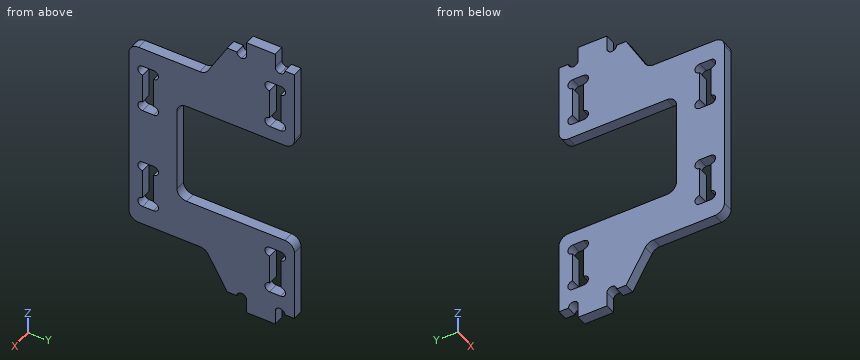
from build123d import *

# Parameters (mm, degrees)
EXTRUDE_1_DEPTH = 2.2
FILLET_1_R      = 2


with BuildPart() as part:
    # 草图1 → 凸台-拉伸1 (new body)
    with BuildSketch(Plane(origin=(0, 0, 0), x_dir=(0, 0, -1), z_dir=(1, 0, 0))):
        with BuildLine():
            Line((-20.1, -17.25), (20.1, -17.25))
            Line((20.1, -17.25), (20.1, -1.311067127))
            Line((20.1, -1.311067127), (28, 3.25))
            Line((28, 3.25), (28, 5.24))
            ThreePointArc((28, 5.24), (26.995, 6.245), (28, 7.25))
            Line((28, 7.25), (31, 7.25))
            Line((31, 7.25), (31, 13.25))
            Line((31, 13.25), (28, 13.25))
            ThreePointArc((28, 13.25), (26.995, 14.255), (28, 15.26))
            Line((28, 15.26), (28, 17.25))
            Line((28, 17.25), (10.9, 17.25))
            Line((10.9, 17.25), (10.9, -7.25))
            Line((10.9, -7.25), (-10.9, -7.25))
            Line((-10.9, -7.25), (-10.9, 17.25))
            Line((-10.9, 17.25), (-28, 17.25))
            Line((-28, 17.25), (-28, 15.26))
            ThreePointArc((-28, 15.26), (-27.289357685, 14.965642315), (-26.995, 14.255))
            ThreePointArc((-26.995, 14.255), (-27.289357685, 13.544357685), (-28, 13.25))
            Line((-28, 13.25), (-31, 13.25))
            Line((-31, 13.25), (-31, 7.25))
            Line((-31, 7.25), (-28, 7.25))
            ThreePointArc((-28, 7.25), (-27.289357685, 6.955642315), (-26.995, 6.245))
            ThreePointArc((-26.995, 6.245), (-27.289357685, 5.534357685), (-28, 5.24))
            Line((-28, 5.24), (-28, 3.25))
            Line((-28, 3.25), (-20.1, -1.311067127))
            Line((-20.1, -1.311067127), (-20.1, -17.25))
        make_face()
        with BuildLine():
            Line((-7.91, -14.4), (-14.09, -14.4))
            ThreePointArc((-14.09, -14.4), (-15.095, -15.405), (-16.1, -14.4))
            Line((-16.1, -14.4), (-16.1, -12.1))
            ThreePointArc((-16.1, -12.1), (-15.095, -11.095), (-14.09, -12.1))
            Line((-14.09, -12.1), (-7.91, -12.1))
            ThreePointArc((-7.91, -12.1), (-6.905, -11.095), (-5.9, -12.1))
            Line((-5.9, -12.1), (-5.9, -14.4))
            ThreePointArc((-5.9, -14.4), (-6.905, -15.405), (-7.91, -14.4))
        make_face(mode=Mode.SUBTRACT)
        with BuildLine():
            Line((16.1, -12.1), (16.1, -14.4))
            ThreePointArc((16.1, -14.4), (15.095, -15.405), (14.09, -14.4))
            Line((14.09, -14.4), (7.91, -14.4))
            ThreePointArc((7.91, -14.4), (6.905, -15.405), (5.9, -14.4))
            Line((5.9, -14.4), (5.9, -12.1))
            ThreePointArc((5.9, -12.1), (6.905, -11.095), (7.91, -12.1))
            Line((7.91, -12.1), (14.09, -12.1))
            ThreePointArc((14.09, -12.1), (15.095, -11.095), (16.1, -12.1))
        make_face(mode=Mode.SUBTRACT)
        with BuildLine():
            Line((-15.91, 12.1), (-22.09, 12.1))
            ThreePointArc((-22.09, 12.1), (-23.095, 11.095), (-24.1, 12.1))
            Line((-24.1, 12.1), (-24.1, 14.4))
            ThreePointArc((-24.1, 14.4), (-23.095, 15.405), (-22.09, 14.4))
            Line((-22.09, 14.4), (-15.91, 14.4))
            ThreePointArc((-15.91, 14.4), (-14.905, 15.405), (-13.9, 14.4))
            Line((-13.9, 14.4), (-13.9, 12.1))
            ThreePointArc((-13.9, 12.1), (-14.905, 11.095), (-15.91, 12.1))
        make_face(mode=Mode.SUBTRACT)
        with BuildLine():
            Line((13.9, 12.1), (13.9, 14.4))
            ThreePointArc((13.9, 14.4), (14.905, 15.405), (15.91, 14.4))
            Line((15.91, 14.4), (22.09, 14.4))
            ThreePointArc((22.09, 14.4), (23.095, 15.405), (24.1, 14.4))
            Line((24.1, 14.4), (24.1, 12.1))
            ThreePointArc((24.1, 12.1), (23.095, 11.095), (22.09, 12.1))
            Line((22.09, 12.1), (15.91, 12.1))
            ThreePointArc((15.91, 12.1), (14.905, 11.095), (13.9, 12.1))
        make_face(mode=Mode.SUBTRACT)
    extrude(amount=EXTRUDE_1_DEPTH)

    # 圆角1
    fillet_1_edges = [part.edges().sort_by_distance(p)[0] for p in [
        (1.1, -1.311067127, -20.1),
        (1.1, -17.25, -20.1),
        (1.1, -17.25, 20.1),
        (1.1, -1.311067127, 20.1),
        (1.1, 17.25, 10.9),
        (1.1, -7.25, 10.9),
        (1.1, -7.25, -10.9),
        (1.1, 17.25, -10.9),
    ]]
    fillet(fillet_1_edges, radius=FILLET_1_R)


solid = part.part
Could you check a few things on this model? Use its own coordinates, in mm. Round coordinates to 2 decimals unless told otherwise and drop trailing zeros. Write each loop counter-clockwise with the first axis right and the second up, starting at its lowest first coordinate (ties: lowest second). Pieces come first, ordered by that corner, then holes. Notation, with made-up numbers: (-24.5, 82.25) - (11.5, 82.25) arc R27 cw to (11.5, 107.25) - close; hole circle Ø1 at (13.25, -30.75). An arc over 180 degrees is marked (long way). Put each result on its own line as item: value. Start each with the question number.
(1) I need wall thicknesses on probe 1 along Y at (x, z) = (2.05, -15); probe 2 along Y at (x, z) = (1.95, 13); probe 3 along Z at (x, y) = (1.25, 5). Which ranges of each line are inside material? Lowest first, please.
(2) I want a section at B-B, the plane z = 17. Please give me the cut outline in (x, y), plus the area to 3 significant figures.
(3) I want a section at A-A, the plane y = -13. Please give me the cut outline in (x, z), plus the area to 3 significant figures.
(4) I want a section at C-C, the plane y = 2. Please give me the cut outline in (x, z).
(5) Will these pins go through, and if not, where does the flat tip stop? pin 1 (1.1 mm diameter, centred on x = 1, z = -29, fed in from +Y); pin 2 (1 mm diameter, centred on x = 2, y = -12.5, fed in from -Z); pin 3 (0.7 mm diameter, centred on x = 1, z = 9.5, fed in from +Y).
(6) I want a section at D-D, the plane x = 1.6. Give the number of separate pieces and of enclosed holes in the cut face, plus the area to 3 significant figures.
Here are the results:
1. probe 1: y = -17.25 to -15.4, -11.1 to 11.1, 15.4 to 17.25
1. probe 2: y = -17.25 to -14.4, -12.1 to 17.25
1. probe 3: z = -28 to -10.9, 10.9 to 28
2. outline: (0, -17.25) - (2.2, -17.25) - (2.2, 12.1) - (0, 12.1) - close; (0, 14.4) - (2.2, 14.4) - (2.2, 17.25) - (0, 17.25) - close
2. area: 70.8 mm^2
3. outline: (0, -20.1) - (2.2, -20.1) - (2.2, -16.1) - (0, -16.1) - close; (0, -5.9) - (2.2, -5.9) - (2.2, 5.9) - (0, 5.9) - close; (0, 16.1) - (2.2, 16.1) - (2.2, 20.1) - (0, 20.1) - close
3. area: 43.6 mm^2
4. outline: (0, -25.83) - (2.2, -25.83) - (2.2, -10.9) - (0, -10.9) - close; (0, 10.9) - (2.2, 10.9) - (2.2, 25.83) - (0, 25.83) - close
5. pin 1: stops at y = 13.25
5. pin 2: stops at z = -20.1
5. pin 3: stops at y = -7.01
6. separate pieces: 1
6. enclosed holes: 4
6. area: 1,020 mm^2
